Can you work these out from the model? Positions are in its coordinate system, mm. Coordinates: 2 decimals unless noted, no trailing zeros. Loops run counter-clockwise (first coordinate to the right, second up) from the corner with the lowest first, then second, coordinate; pieces in that order, holes last. Notation, with made-up numbers: M 76.5,-32.5 L 118.5,-32.5 A33 cw 118.5,-4.5 Z; hole C 37.5,8 d4. An arc over 180 degrees is marked long. Answer as a JSON object with one key per item and string values. Group by question number.
Item 1: We'd pull the mould along Z, two halves only. Please class faces 1 (the flat face through (62.31, 1.48, -4.23)), 2 (the flat face through (112, 0, 1)): +Z half, -Z half, draft (parallel to the pull), parting line (faces both ways), or undercut.
Item 2: Suppose I cut it at C-C (x = 54). Write out the boundary of the cut face in (y, z).
Item 3: Suppose I cut it at B-B (z = -30). Write out the boundary of the cut face in (x, y), then the cut area to 3 significant figures.
Item 4: If I drill on line 1 (Z direction, x = 208.5, y = 2); line 2 (Z direction, x = 203.5, y = 2.1); line 3 (X direction, y = 0.9, z = -17.5), over which ranges is the centre line in solid material (lowest first)?
Item 5: Suppose I cut it at D-D (y = 0.7). Count the separate pieces of the cut face and the enclosed holes in it, then the cut area to 3 significant figures.
Item 6: Suppose I cut it at A-A (x = 104.25). Write out the boundary of the cut face in (y, z), then the cut area to 3 significant figures.
Item 7: I'm going to push flat-ended pins straight in: pin 1 Ø0.9 at (x, y) = (60.5, 2) entering from +Z; pin 2 Ø1 at (x, y) = (164, 1.5) entering from -Z; pin 3 Ø5 at (x, z) = (129.36, 5.75) entering from +Y; pin 4 Ø1.5 at (y, z) = (2, 12.5) entering from +X. Where does each tip first touch, or does it pass through?
```python
from build123d import *

# Parameters (mm, degrees)
SKETCH_2_R      = 1.7
SKETCH_2_R_2    = 11.15
SKETCH_2_R_3    = 4
SKETCH_2_R_4    = 2.15
EXTRUDE_1_DEPTH = 3


with BuildPart() as part:
    # 草图2 → 凸台-拉伸1 (new body)
    with BuildSketch(Plane(origin=(0, 0, 0), x_dir=(1, 0, 0), z_dir=(0, 1, 0))):
        with BuildLine():
            Line((-3.5, -3.5), (69.783530787, -3.5))
            ThreePointArc((69.783530787, -3.5), (72.878191201, -4.359661789), (75.086064512, -6.692307692))
            ThreePointArc((75.086064512, -6.692307692), (104.25, -24.25), (133.413935488, -6.692307692))
            ThreePointArc((133.413935488, -6.692307692), (135.621808799, -4.359661789), (138.716469213, -3.5))
            Line((138.716469213, -3.5), (212, -3.5))
            Line((212, -3.5), (212, 21))
            Line((212, 21), (138.716469213, 21))
            ThreePointArc((138.716469213, 21), (135.621808799, 21.859661789), (133.413935488, 24.192307692))
            ThreePointArc((133.413935488, 24.192307692), (104.25, 41.75), (75.086064512, 24.192307692))
            ThreePointArc((75.086064512, 24.192307692), (72.878191201, 21.859661789), (69.783530787, 21))
            Line((69.783530787, 21), (-3.5, 21))
            Line((-3.5, 21), (-3.5, -3.5))
        make_face()
        with Locations(Location((0, 17.5, 0), (0, 0, 270))):
            Circle(SKETCH_2_R, mode=Mode.SUBTRACT)
        with Locations(Location((23.5, 17.5, 0), (0, 0, 270))):
            Circle(SKETCH_2_R, mode=Mode.SUBTRACT)
        with Locations(Location((0, 0, 0), (0, 0, 270))):
            Circle(SKETCH_2_R, mode=Mode.SUBTRACT)
        with Locations(Location((23.5, 0, 0), (0, 0, 270))):
            Circle(SKETCH_2_R, mode=Mode.SUBTRACT)
        with Locations(Location((104.25, 8.75, 0), (0, 0, 270))):
            Circle(SKETCH_2_R_2, mode=Mode.SUBTRACT)
        with Locations(Location((104.25, 28, 0), (0, 0, 270))):
            Circle(SKETCH_2_R_3, mode=Mode.SUBTRACT)
        with Locations(Location((104.25, 37.75, 0), (0, 0, 270))):
            Circle(SKETCH_2_R_4, mode=Mode.SUBTRACT)
        with Locations(Location((185, 0, 0), (0, 0, 90))):
            Circle(SKETCH_2_R, mode=Mode.SUBTRACT)
        with Locations(Location((208.5, 0, 0), (0, 0, 90))):
            Circle(SKETCH_2_R, mode=Mode.SUBTRACT)
        with Locations(Location((208.5, 17.5, 0), (0, 0, 90))):
            Circle(SKETCH_2_R, mode=Mode.SUBTRACT)
        with Locations(Location((185, 17.5, 0), (0, 0, 90))):
            Circle(SKETCH_2_R, mode=Mode.SUBTRACT)
        with Locations(Location((129.36473671, -5.75, 0), (0, 0, 270))):
            Circle(SKETCH_2_R_4, mode=Mode.SUBTRACT)
        with Locations(Location((79.13526329, -5.75, 0), (0, 0, 270))):
            Circle(SKETCH_2_R_4, mode=Mode.SUBTRACT)
        Polygon((4.525728913, 16), (18.974271087, 16), (11.75, 10.620223658), align=None, mode=Mode.SUBTRACT)
        Polygon((1.5, 14.512755065), (1.5, 2.987244935), (9.238556802, 8.75), align=None, mode=Mode.SUBTRACT)
        Polygon((189.525728913, 16), (196.75, 10.620223658), (203.974271087, 16), align=None, mode=Mode.SUBTRACT)
        Polygon((207, 2.987244935), (199.261443198, 8.75), (207, 14.512755065), align=None, mode=Mode.SUBTRACT)
        Polygon((14.261443198, 8.75), (22, 2.987244935), (22, 14.512755065), align=None, mode=Mode.SUBTRACT)
        Polygon((11.75, 6.879776342), (18.974271087, 1.5), (4.525728913, 1.5), align=None, mode=Mode.SUBTRACT)
        Polygon((42.474271087, 1.5), (28.025728913, 1.5), (35.25, 6.879776342), align=None, mode=Mode.SUBTRACT)
        Polygon((32.738556802, 8.75), (25, 14.512755065), (25, 2.987244935), align=None, mode=Mode.SUBTRACT)
        Polygon((35.25, 10.620223658), (28.025728913, 16), (42.474271087, 16), align=None, mode=Mode.SUBTRACT)
        Polygon((45.5, 14.512755065), (37.761443198, 8.75), (45.5, 2.987244935), align=None, mode=Mode.SUBTRACT)
        Polygon((51.525728913, 16), (65.974271087, 16), (58.75, 10.620223658), align=None, mode=Mode.SUBTRACT)
        Polygon((51.525728913, 1.5), (58.75, 6.879776342), (65.974271087, 1.5), align=None, mode=Mode.SUBTRACT)
        Polygon((61.261443198, 8.75), (69, 2.987244935), (69, 14.512755065), align=None, mode=Mode.SUBTRACT)
        Polygon((56.238556802, 8.75), (48.5, 14.512755065), (48.5, 2.987244935), align=None, mode=Mode.SUBTRACT)
        Polygon((142.525728913, 1.5), (156.974271087, 1.5), (149.75, 6.879776342), align=None, mode=Mode.SUBTRACT)
        Polygon((139.5, 14.512755065), (147.238556802, 8.75), (139.5, 2.987244935), align=None, mode=Mode.SUBTRACT)
        Polygon((149.75, 10.620223658), (156.974271087, 16), (142.525728913, 16), align=None, mode=Mode.SUBTRACT)
        Polygon((160, 2.987244935), (152.261443198, 8.75), (160, 14.512755065), align=None, mode=Mode.SUBTRACT)
        Polygon((173.25, 6.879776342), (166.025728913, 1.5), (180.474271087, 1.5), align=None, mode=Mode.SUBTRACT)
        Polygon((163, 2.987244935), (163, 14.512755065), (170.738556802, 8.75), align=None, mode=Mode.SUBTRACT)
        Polygon((166.025728913, 16), (173.25, 10.620223658), (180.474271087, 16), align=None, mode=Mode.SUBTRACT)
        Polygon((183.5, 2.987244935), (175.761443198, 8.75), (183.5, 14.512755065), align=None, mode=Mode.SUBTRACT)
        Polygon((186.5, 2.987244935), (186.5, 14.512755065), (194.238556802, 8.75), align=None, mode=Mode.SUBTRACT)
        Polygon((189.525728913, 1.5), (203.974271087, 1.5), (196.75, 6.879776342), align=None, mode=Mode.SUBTRACT)
    extrude(amount=EXTRUDE_1_DEPTH)


solid = part.part
```
From the geometry:
{
 "1": {"face 1": "undercut", "face 2": "draft"},
 "2": {"outline": "M 0,-21 L 3,-21 L 3,-16 L 0,-16 Z; M 0,-14.16 L 3,-14.16 L 3,-10.42 L 0,-10.42 Z; M 0,-7.08 L 3,-7.08 L 3,-3.34 L 0,-3.34 Z; M 0,-1.5 L 3,-1.5 L 3,3.5 L 0,3.5 Z"},
 "3": {"outline": "M 79,0 L 100.79,0 L 100.79,3 L 79,3 Z; M 107.71,0 L 129.5,0 L 129.5,3 L 107.71,3 Z", "area": "131 mm2"},
 "4": {"line 1": "-21 to -19.2, -15.8 to -1.7, 1.7 to 3.5", "line 2": "-21 to -16, -15.65 to -11.91, -5.59 to -1.85, -1.5 to 3.5", "line 3": "-3.5 to -1.7, 1.7 to 21.8, 25.2 to 97.34, 111.16 to 183.3, 186.7 to 206.8, 210.2 to 212"},
 "5": {"separate pieces": "1", "enclosed holes": "37", "area": "5,570 mm2"},
 "6": {"outline": "M 0,-41.75 L 3,-41.75 L 3,-39.9 L 0,-39.9 Z; M 0,-35.6 L 3,-35.6 L 3,-32 L 0,-32 Z; M 0,-24 L 3,-24 L 3,-19.9 L 0,-19.9 Z; M 0,2.4 L 3,2.4 L 3,24.25 L 0,24.25 Z", "area": "94.2 mm2"},
 "7": {"pin 1": "z = 3.5", "pin 2": "z = -21", "pin 3": "y = 3", "pin 4": "x = 130.11"}
}
